For this review, take the finished solid that the model builds, in its own axes (mm). Face numbers are marked on the shaded views. A direction names the side the tool comes from. Coordinates: 2 decimals unless noted, no trailing zeros. Write each loop counter-clockwise with the first axis right and the second up, starting at its lowest first coordinate (ties: lowest second). Pieces come first, ordered by that corner, then holes. Notation, with made-up numbers: M -30,8 L 7,8 A26 ccw 7,28 Z; hole C 30,16 d1. An arc over 180 degrees is marked long. One line per question, with ' | ' between items.
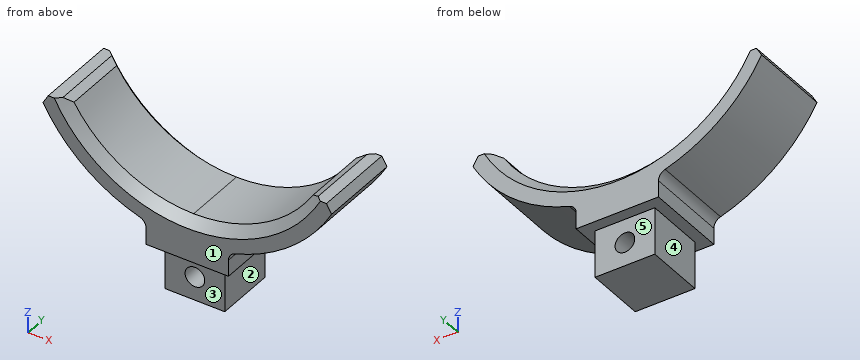
from build123d import *

# Parameters (mm, degrees)
F0_W        = 16.129
F0_H        = 25.4
F1_DEPTH    = 44.45
F2_W        = 32.258
F2_H        = 6.096
F3_DEPTH    = 25.4
F4_R        = 5.30225
F5_DEPTH    = 38.355
F6_R        = 5.08
F7_T1_DEPTH = 59.6994752683
F7_T4_ANGLE = 139.6602442287
F7_T6_ANGLE = 139.6602442287
F8_T1_DEPTH = 71.752763855


# Not quite as in the source:
# - a fillet or chamfer that OpenCascade refuses, or shapes differently, is made with other operations: its cross-section is extruded or revolved along the edge and cut away or added


with BuildPart() as f1:
    # F0 (on Front) → F1 (new body)
    with BuildSketch(Plane.XZ):
        with BuildLine():
            ThreePointArc((0, -76.2), (-38.1, -65.9911357684), (-65.9911357684, -38.1))
            Line((-65.9911357684, -38.1), (-80.3218525683, -38.1))
            ThreePointArc((-80.3218525683, -38.1), (-56.6075409411, -68.5477666201), (-22.225, -86.0770548695))
            Line((-22.225, -86.0770548695), (0, -86.0770548695))
            Line((0, -86.0770548695), (0, -76.2))
        make_face()
        with BuildLine():
            Line((80.3218525683, -38.1), (65.9911357684, -38.1))
            ThreePointArc((65.9911357684, -38.1), (38.1, -65.9911357684), (0, -76.2))
            Line((0, -76.2), (0, -86.0770548695))
            Line((0, -86.0770548695), (22.225, -86.0770548695))
            ThreePointArc((22.225, -86.0770548695), (56.6075409411, -68.5477666201), (80.3218525683, -38.1))
        make_face()
        with BuildLine():
            Line((22.225, -98.7770548695), (22.225, -86.0770548695))
            ThreePointArc((22.225, -86.0770548695), (11.2017816017, -88.1914399982), (0, -88.9))
            Line((0, -88.9), (0, -98.7770548695))
            Line((0, -98.7770548695), (16.129, -98.7770548695))
            Line((16.129, -98.7770548695), (22.225, -98.7770548695))
        make_face()
        with BuildLine():
            ThreePointArc((0, -88.9), (-11.2017816017, -88.1914399982), (-22.225, -86.0770548695))
            Line((-22.225, -86.0770548695), (-22.225, -98.7770548695))
            Line((-22.225, -98.7770548695), (-16.129, -98.7770548695))
            Line((-16.129, -98.7770548695), (0, -98.7770548695))
            Line((0, -98.7770548695), (0, -88.9))
        make_face()
        with Locations((8.0645, -111.4770548695)):
            Rectangle(F0_W, F0_H)
        with Locations((-8.0645, -111.4770548695)):
            Rectangle(F0_W, F0_H)
        with BuildLine():
            Line((22.225, -86.0770548695), (0, -86.0770548695))
            Line((0, -86.0770548695), (0, -88.9))
            ThreePointArc((0, -88.9), (11.2017816017, -88.1914399982), (22.225, -86.0770548695))
        make_face()
        with BuildLine():
            Line((0, -88.9), (0, -86.0770548695))
            Line((0, -86.0770548695), (-22.225, -86.0770548695))
            ThreePointArc((-22.225, -86.0770548695), (-11.2017816017, -88.1914399982), (0, -88.9))
        make_face()
    extrude(amount=F1_DEPTH)

    # F2 (on face) → F3 (cut)
    with BuildSketch(Plane(origin=(0, 0, -124.1770548695), x_dir=(1, 0, 0), z_dir=(0, 0, -1))):
        with Locations((0, 41.402)):
            Rectangle(F2_W, F2_H)
        with Locations((0, 3.048)):
            Rectangle(F2_W, F2_H)
    extrude(amount=-F3_DEPTH, mode=Mode.SUBTRACT)

    # F4 (on face) → F5 (cut, through all)
    with BuildSketch(Plane.XZ.offset(38.354)):
        with Locations((0, -111.4770548695)):
            Circle(F4_R)
    extrude(amount=-F5_DEPTH, mode=Mode.SUBTRACT)

    # F6
    f6_edges = [f1.edges().sort_by_distance(p)[0] for p in [
        (-22.225, -22.225, -86.077055),
        (22.225, -22.225, -86.077055),
    ]]
    fillet(f6_edges, radius=F6_R)

    # F7: chamfer of 5.08 on 4 edges, made by hand

    # F7_s2 → F7_t1 (cut)
    with BuildSketch(Plane.XZ.offset(-7.6247376341)):
        with BuildLine():
            Line((-68.8616438956, -38.1), (-64.5577911521, -40.48125))
            ThreePointArc((-64.5577911521, -40.48125), (-65.2398633811, -39.3725821609), (-65.9911357684, -38.1))
            Line((-65.9911357684, -38.1), (-68.8616438956, -38.1))
        make_face()
        with BuildLine():
            Line((64.5577911521, -40.48125), (68.8616438956, -38.1))
            Line((68.8616438956, -38.1), (65.9911357684, -38.1))
            ThreePointArc((65.9911357684, -38.1), (65.2398633811, -39.3725821609), (64.5577911521, -40.48125))
        make_face()
    extrude(amount=F7_T1_DEPTH, mode=Mode.SUBTRACT)

    # F7_s3 → F7_t4 (revolve, cut)
    with BuildSketch(Plane(origin=(0, 0, 0), x_dir=(0, 1, 0), z_dir=(0.3448047573, 0, 0.9386744267))):
        Polygon((-44.45, -81.28), (-39.37, -76.2), (-44.45, -76.2), align=None)
    revolve(axis=Axis((0, -44.45, 0), (0, 1, 0)), revolution_arc=F7_T4_ANGLE, mode=Mode.SUBTRACT)

    # F7_s5 → F7_t6 (revolve, cut)
    with BuildSketch(Plane(origin=(0, 0, 0), x_dir=(0, 1, 0), z_dir=(0.3448047573, 0, 0.9386744267))):
        Polygon((0, -81.28), (-5.08, -76.2), (0, -76.2), align=None)
    revolve(axis=Axis((0, 0, 0), (0, 1, 0)), revolution_arc=F7_T6_ANGLE, mode=Mode.SUBTRACT)

    # F8: chamfer of 5.08 on 2 edges, made by hand

    # F8_s2 → F8_t1 (cut)
    with BuildSketch(Plane.XZ.offset(-13.6513819275)):
        with BuildLine():
            Line((74.966768006, -37.9250746392), (77.988352908, -43.0368427057))
            Line((77.988352908, -43.0368427057), (78.0773642839, -43.0858277541))
            ThreePointArc((78.0773642839, -43.0858277541), (79.2049019091, -40.5939443284), (80.4136489712, -38.1435428571))
            Line((80.4136489712, -38.1435428571), (80.3218525683, -37.9984))
            ThreePointArc((80.3218525683, -37.9984), (77.6443102871, -37.9984), (74.966768006, -37.8234746392))
            Line((74.966768006, -37.8234746392), (74.966768006, -37.9250746392))
        make_face()
        with BuildLine():
            Line((-77.988352908, -43.0368427057), (-74.966768006, -37.9250746392))
            Line((-74.966768006, -37.9250746392), (-74.966768006, -37.8234746392))
            ThreePointArc((-74.966768006, -37.8234746392), (-77.6443102871, -37.9984), (-80.3218525683, -37.9984))
            Line((-80.3218525683, -37.9984), (-80.4136489712, -38.1435428571))
            ThreePointArc((-80.4136489712, -38.1435428571), (-79.2049019091, -40.5939443284), (-78.0773642839, -43.0858277541))
            Line((-78.0773642839, -43.0858277541), (-77.988352908, -43.0368427057))
        make_face()
    extrude(amount=F8_T1_DEPTH, mode=Mode.SUBTRACT)


solid = f1.part
1. Machinability: for the marked faces 1, 2, 3, 4 and 5, which of the approach directions +Z, -Z, +X, -X, +Y, -Y give a long, thin tool a straight path to every point of the face, cutting with its end or side? Answer none if there is none.
Computed values:
face 1: +Z, -Z, +X, -X, -Y | face 2: -Z, +X, +Y, -Y | face 3: -Z, +X, -X, -Y | face 4: -Z, -X, +Y, -Y | face 5: -Z, +X, -X, +Y
2. For line 1 along X through (y, z) = (-12.5, -111); line 2 along X through (y, z) = (-39.5, -91.5) (3 decimals); line 3 along X through (y, z) = (-31.5, -104), list the stretches that pass through material, from the lowest coordinate up.
Computed values:
line 1: x = -16.13 to -5.28, 5.28 to 16.13 | line 2: x = -22.225 to 22.225 | line 3: x = -16.13 to 16.13
3. Clearance check with flat-ended pins moving along their axes: P1, Ø7.5, axis at y = -15.5, z = -112.5, coming from the -X side; P2, Ø1.5, axis at x = -50.5, y = -32, coming from the -Z side; P3, Ø10, axis at y = -6, z = -100, coming from the +X side (3 decimals); P4, Ø12, axis at x = 19.5, z = -101.5, coming from the -Y side. State where each tip first meets the part, or that it passes through.
Computed values:
P1: stops at x = -16.13 | P2: stops at z = -73.68 | P3: stops at x = 22.225 | P4: stops at y = -44.45
4. Take a section at A-A on y = -25. State the section outline as (x, z) points (1 decimal).
Computed values:
outline: M -77.9,-42.9 A88.9 ccw -25.8,-85.1 A5.1 cw -22.2,-89.9 L -22.2,-98.8 L -16.1,-98.8 L -16.1,-124.2 L 16.1,-124.2 L 16.1,-98.8 L 22.2,-98.8 L 22.2,-89.9 A5.1 cw 25.8,-85.1 A88.9 ccw 77.9,-42.9 L 75.1,-38.1 L 68.9,-38.1 L 64.6,-40.5 A76.2 cw -64.6,-40.5 L -68.9,-38.1 L -75.1,-38.1 Z; hole C 0,-111.5 d10.6
